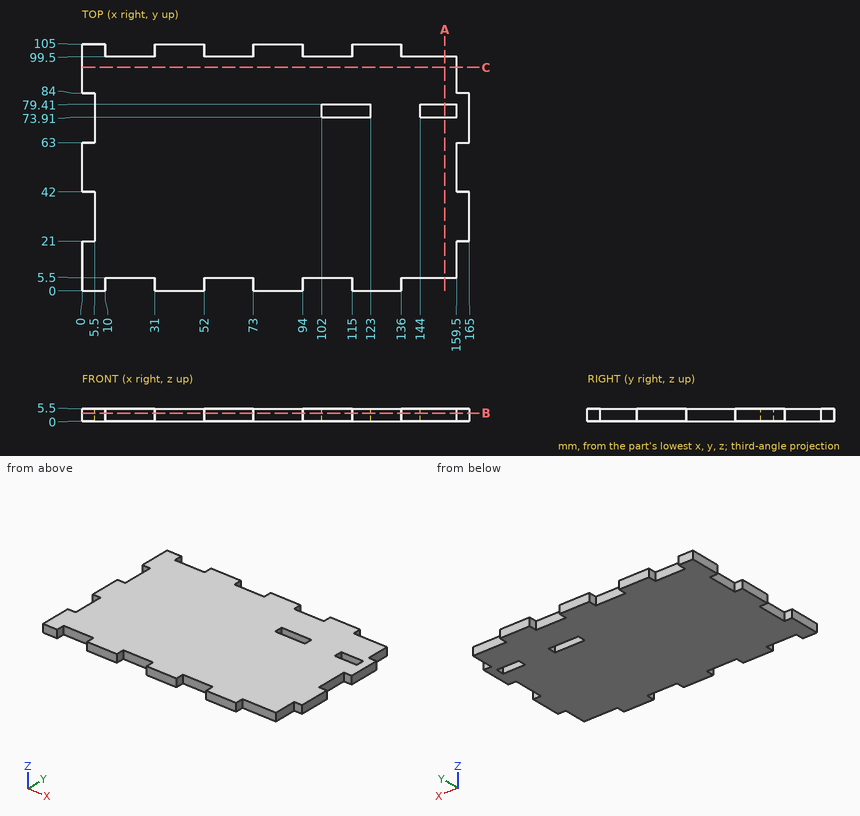
Input: dimensioned drawing with shaded views. Units: mm. Origin: part minimum x, y, z. Coordinates: 2 decimals unless noted, no trailing zeros. Loops run counter-clockwise (first coordinate to the right, second up) from the corner with the lowest first, then second, coordinate; pieces in that order, holes last. Notation, with made-up numbers: M 60,42 L 78,42 A5 cw 78,50 Z; hole C -25.75,86 d10. An arc over 180 degrees is marked long. Put each result on its own line as item: value.
(1) Cut plane A-A on x = 154.5. Return the cut outline in (y, z), then the cut area to 3 significant figures.
Answer sheet:
outline: M 5.5,0 L 73.91,0 L 73.91,5.5 L 5.5,5.5 Z; M 79.41,0 L 99.5,0 L 99.5,5.5 L 79.41,5.5 Z
area: 487 mm^2
(2) Cut plane B-B on z = 3.55. State how many separate pieces and enclosed holes the cut face has, then the cut area to 3 significant figures.
Answer sheet:
separate pieces: 1
enclosed holes: 2
area: 15,600 mm^2
(3) Cut plane C-C on y = 95. Return the cut outline in (x, z).
Answer sheet:
outline: M 0,0 L 159.5,0 L 159.5,5.5 L 0,5.5 Z
(4) Material intervals for probe 1 along Y at (x, z) = (118.5, 0.4); probe 2 along Y at (x, z) = (157.5, 0.85); probe 3 along X at (y, z) = (30, 5.1), sorted ascending.
Answer sheet:
probe 1: y = 0 to 73.91, 79.41 to 105
probe 2: y = 5.5 to 73.91, 79.41 to 99.5
probe 3: x = 5.5 to 165
(5) First-contact query: pin 1 (3 mm diameter, centred on y = 101.5, z = 4, fed in from +X); pin 2 (3 mm diameter, centred on x = 101, z = 3, fed in from +Y); pin 3 (3 mm diameter, centred on y = 76.5, z = 2.5, fed in from -X). Flat tips, straight axial feed; report the tip coordinate or a pass-through.
Answer sheet:
pin 1: stops at x = 136
pin 2: stops at y = 99.5
pin 3: stops at x = 5.5
